from build123d import *

# Parameters (mm, degrees)
F1_DEPTH = 133.35
F2_R     = 4.5466
F3_DEPTH = 25.4
F4_R     = 4.5466
F5_DEPTH = 25.4
F6_R     = 6.35


with BuildPart() as f1:
    # F0 (on Front) → F1 (new body)
    with BuildSketch(Plane.XZ):
        Polygon((-40.797278, 26.517693), (-40.797278, -11.582307), (-34.447278, -11.582307), (-34.447278, 20.167693), (3.652722, 20.167693), (3.652722, 26.517693), align=None)
    extrude(amount=F1_DEPTH)

    # F2 (on face) → F3 (cut)
    with BuildSketch(Plane(origin=(-40.797278, 0, 0), x_dir=(0, -1, 0), z_dir=(-1, 0, 0))):
        with Locations((107.95, -0.482507)):
            Circle(F2_R)
        with Locations((44.45, -0.482507)):
            Circle(F2_R)
    extrude(amount=-F3_DEPTH, mode=Mode.SUBTRACT)

    # F4 (on face) → F5 (cut)
    with BuildSketch(Plane.XY.offset(26.517693)):
        with Locations((-9.047278, -12.7)):
            Circle(F4_R)
        with Locations((-9.047278, -114.3)):
            Circle(F4_R)
    extrude(amount=-F5_DEPTH, mode=Mode.SUBTRACT)

    # F6
    f6_edges = [f1.edges().sort_by_distance(p)[0] for p in [
        (3.652722, 0, 23.342693),
        (-37.622278, 0, -11.582307),
        (3.652722, -133.35, 23.342693),
        (-37.622278, -133.35, -11.582307),
    ]]
    fillet(f6_edges, radius=F6_R)


solid = f1.part
Can you work these out from the model? Positions are in its coordinate system, mm. A direction names the side the tool comes from. Give positions to 0.01 mm unless a question says otherwise; leave off trailing zeros. Order: outer loops, then holes, each group sorted by start corner. A loop starts at its lowest first (then second) coordinate and runs counter-clockwise, first axis right, second up. Notation, with made-up numbers: (69.25, 76) - (80.25, 76) arc R25 cw to (80.25, 97) - close; hole circle Ø5 at (4, 31). An arc over 180 degrees is marked (long way). Write each question's results on one line, items separated by ' | '.
1) Suppose I cut it at A-A, the plane y = -12.7. Write out the boundary of the cut face in (x, z), then the cut area to 3 significant figures.
Final values:
outline: (-40.8, -11.58) - (-34.45, -11.58) - (-34.45, 20.17) - (-13.59, 20.17) - (-13.59, 26.52) - (-40.8, 26.52) - close; (-4.5, 20.17) - (3.65, 20.17) - (3.65, 26.52) - (-4.5, 26.52) - close | area: 426 mm^2
2) Suppose I cut it at C-C, the plane x = -23.5. Write out the boundary of the cut face in (y, z).
Final values:
outline: (-133.35, 20.17) - (0, 20.17) - (0, 26.52) - (-133.35, 26.52) - close
3) Suppose I cut it at D-D, the plane y = -41.5. Write out the boundary of the cut face in (x, z).
Final values:
outline: (-40.8, -11.58) - (-34.45, -11.58) - (-34.45, -3.94) - (-40.8, -3.94) - close; (-40.8, 2.98) - (-34.45, 2.98) - (-34.45, 20.17) - (3.65, 20.17) - (3.65, 26.52) - (-40.8, 26.52) - close
4) Please list where these lines run through material, in increasing order: line 1 along Z through (x, y) = (-36.75, -107.95); line 2 along Y through (x, z) = (-36.5, -2.5); line 3 along Z through (x, y) = (-16.5, -83). Write a range as [from, to].
Final values:
line 1: z = [-11.58, -5.03], [4.06, 26.52] | line 2: y = [-133.35, -112.02], [-103.88, -48.52], [-40.38, 0] | line 3: z = [20.17, 26.52]
5) If we mould it in two halves opening along Y, with no side actions, what happens to faces 3 (the face through (-40.797, -66, 8)), 4 (the face through (-9.639, -109.792, 23.387)), 5 (the face through (1.74, -131.54, 23.39)), 6 (the face through (-37.667, -39.908, -0.283))? For each: pulls with the +Y half, pulls with the -Y half, needs draft (parallel to the pull), parting line crosses it, or undercut.
Final values:
face 3: needs draft | face 4: undercut | face 5: pulls with the -Y half | face 6: undercut
6) I'm going to push flat-ended pins straight in: pin 1 Ø4 at (y, z) = (-70.5, -6.5) entering from +X; pin 2 Ø12 at (x, y) = (-5, -103.5) entering from -Z. Where does each tip first touch, or does it pass through?
Final values:
pin 1: stops at x = -34.45 | pin 2: stops at z = 20.17
7) Suppose I cut it at B-B, the plane y = -98.5. Write out the boundary of the cut face in (x, z).
Final values:
outline: (-40.8, -11.58) - (-34.45, -11.58) - (-34.45, 20.17) - (3.65, 20.17) - (3.65, 26.52) - (-40.8, 26.52) - close
8) On a 3-axis mill with a long thin cutter (end or side, diameter ignored), from which of +Z, -Z, +X, -X, +Y, -Y can I reach the whole of each face in a straight line? I mean faces 1 (the face through (-16, -66, 20.168)), 2 (the face through (-30, 0, 21)). Say none if no direction works.
Final values:
face 1: -Z, +X, +Y, -Y | face 2: +Z, -Z, +X, -X, +Y
